Source: CAD feature listing. Evaluate the final solid. Frame: model axes, mm. Face numbers are marked on the shaded views. A direction names the side the tool comes from. Coordinates: 2 decimals unless noted, no trailing zeros. Order: outer loops, then holes, each group sorted by start corner. A loop starts at its lowest first (then second) coordinate and runs counter-clockwise, first axis right, second up.
Item 1: Section C-C on y = 41.5. Return the cut outline in (x, z), then the cut area to 3 significant figures.
Item 2: Section B-B on x = 32. Return the cut outline in (y, z).
Item 3: Reachability of the marked faces 1 and 2 from +Z, -Z, +X, -X, +Y, -Y: full face, straight path, thin tool, end or side. Return the list, or none.
Item 4: Ray query, line 1 (Y direction, x = 25, z = 4); line 2 (X direction, y = 8, z = 19.75); line 3 (Z direction, x = 10, y = 42.5). Return the intervals inside material, ascending.
Item 5: Contact query for a flat-ended pin moving along its axis: P1, Ø23, axis at x = 25.5, y = 27, coming from the +Z side. Output: stop coordinate, or through.
Item 6: Mould query, pull axis X, two halves, no side actions, for the marked faces 3, 4 and 5. Classes: released by +X, released by -X, zero draft, split by the parting line, or undercut.
Item 7: Section A-A on z = 4. Return the cut outline in (x, y).
from build123d import *

# Parameters (mm, degrees)
F0_W     = 65.18887
F0_H     = 51.452216
F1_DEPTH = 25.4
F2_T     = -25.4
F3_T     = -2.54
F4_R     = 3.066051


with BuildPart() as f1:
    # F0 (on Top) → F1 (new body)
    with BuildSketch(Plane.XY):
        with Locations((32.594435, 25.726108)):
            Rectangle(F0_W, F0_H)
    extrude(amount=F1_DEPTH)

    # F2
    f2_openings = [f1.faces().sort_by_distance(p)[0] for p in [
        (32.594435, 25.726108, 25.4),
    ]]
    offset(amount=F2_T, openings=f2_openings)

    # F3
    f3_openings = [f1.faces().sort_by_distance(p)[0] for p in [
        (32.594435, 25.726108, 25.4),
    ]]
    offset(amount=F3_T, openings=f3_openings)

    # F4
    f4_edges = [f1.edges().sort_by_distance(p)[0] for p in [
        (0, 0, 12.7),
    ]]
    fillet(f4_edges, radius=F4_R)


solid = f1.part
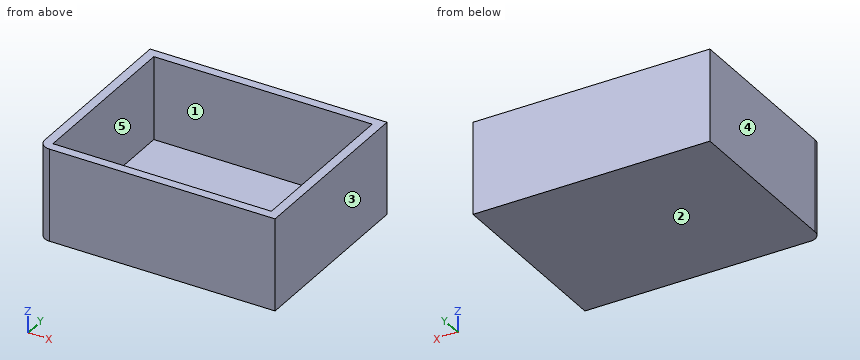
Answer list:
1. outline: (0, 0) - (65.19, 0) - (65.19, 25.4) - (62.65, 25.4) - (62.65, 2.54) - (2.54, 2.54) - (2.54, 25.4) - (0, 25.4) - close
1. area: 282 mm2
2. outline: (0, 0) - (51.45, 0) - (51.45, 25.4) - (48.91, 25.4) - (48.91, 2.54) - (2.54, 2.54) - (2.54, 25.4) - (0, 25.4) - close
3. face 1: +Z
3. face 2: -Z, +X, -X, +Y, -Y
4. line 1: y = 0 to 2.54, 48.91 to 51.45
4. line 2: x = 0 to 2.54, 62.65 to 65.19
4. line 3: z = 0 to 2.54
5. P1: stops at z = 2.54
6. face 3: released by +X
6. face 4: released by -X
6. face 5: undercut
7. outline: (0, 3.07) arc R3.07 ccw to (3.07, 0) - (65.19, 0) - (65.19, 51.45) - (0, 51.45) - close; hole (2.54, 2.54) - (62.65, 2.54) - (62.65, 48.91) - (2.54, 48.91) - close
